The figure shows three views and two pictorial views of one solid part (mm, origin at its lowest corner). Answer the questions. Give positions to 0.01 mm unless a question says otherwise; leave off trailing zeros. Loops run counter-clockwise (first coordinate to the right, second up) from the corner with the lowest first, then second, coordinate; pieces in that order, holes last. Notation, with made-up numbers: (69.25, -13) - (81.25, -13) arc R32 ccw to (81.25, 22) - close; hole circle Ø10 at (-22, 36.25). An arc over 180 degrees is marked (long way). Write item = value, one per line.
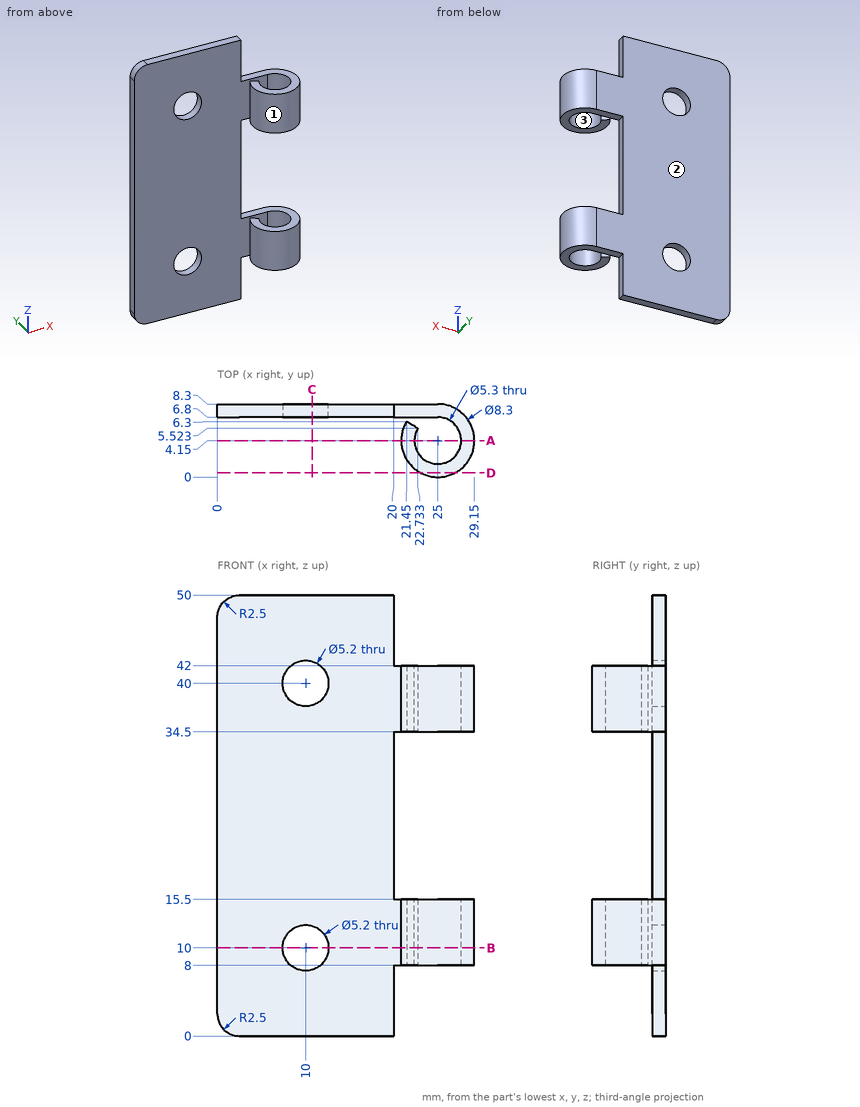
1) A cutting plane is placed at A-A on y = 4.15. Determine the outline of the cut face in (x, z).
Output:
outline = (20.85, 8) - (22.35, 8) - (22.35, 15.5) - (20.85, 15.5) - close; (20.85, 34.5) - (22.35, 34.5) - (22.35, 42) - (20.85, 42) - close; (27.65, 8) - (29.15, 8) - (29.15, 15.5) - (27.65, 15.5) - close; (27.65, 34.5) - (29.15, 34.5) - (29.15, 42) - (27.65, 42) - close
2) A cutting plane is placed at D-D on y = 0.5. Determine the outline of the cut face in (x, z) (1 decimal).
Output:
outline = (23, 8) - (27, 8) - (27, 15.5) - (23, 15.5) - close; (23, 34.5) - (27, 34.5) - (27, 42) - (23, 42) - close
3) A cutting plane is placed at C-C on x = 10.75. Determine the outline of the cut face in (y, z).
Output:
outline = (6.8, 0) - (8.3, 0) - (8.3, 7.51) - (6.8, 7.51) - close; (6.8, 12.49) - (8.3, 12.49) - (8.3, 37.51) - (6.8, 37.51) - close; (6.8, 42.49) - (8.3, 42.49) - (8.3, 50) - (6.8, 50) - close
4) Find the intervals of material crossed by probe 1 along Z at (x, y) = (10, 7.45); probe 2 along X at (y, z) = (4.15, 9.75); probe 3 along Z at (x, y) = (27.5, 6.5), in increasing order.
Output:
probe_1 = 0 to 7.4, 12.6 to 37.4, 42.6 to 50
probe_2 = 20.85 to 22.35, 27.65 to 29.15
probe_3 = 8 to 15.5, 34.5 to 42
5) Each of these flat-tipped pins is pushed along its axis until it touches: P1, Ø5, axis at x = 4, z = 18.5, coming from the -Y side; P2, Ø0.8, axis at y = 7.5, z = 45.5, coming from the +X side; P3, Ø2.5, axis at x = 25, y = 4.5, coming from the -Z side. Where does it stop, or does it pass through?
Output:
P1 = 6.8
P2 = 20
P3 = through
6) The mould has two halves that part along X. Classify the marked faces 1, 2 and 3: pulls with the +X half, pulls with the -X half, needs draft (parallel to the pull), parting line crosses it, or undercut.
Output:
face_1 = parting line crosses it
face_2 = needs draft
face_3 = undercut
7) A cutting plane is placed at B-B on z = 10. Determine the outline of the cut face in (x, y).
Output:
outline = (0, 6.8) - (7.4, 6.8) - (7.4, 8.3) - (0, 8.3) - close; (12.6, 6.8) - (25, 6.8) arc R2.65 cw (long way) to (22.73, 5.52) - (21.45, 6.3) arc R4.15 ccw (long way) to (25, 8.3) - (12.6, 8.3) - close
